Source: CAD feature listing. Evaluate the final solid. Frame: model axes, mm. A direction names the side the tool comes from. Round coordinates to 2 decimals unless told otherwise and drop trailing zeros. Loops run counter-clockwise (first coordinate to the right, second up) from the corner with the lowest first, then second, coordinate; pieces in that order, holes last. Notation, with made-up numbers: (-7, 30.25) - (34, 30.25) arc R11 ccw to (34, 39.25) - close; hole circle Ø6 at (70, -27.5). An arc over 180 degrees is marked (long way). Write item = value, one per line. Start each with the question number.
from build123d import *

# Parameters (mm, degrees)
SKETCH1_R           = 1.25
BOSS_EXTRUDE1_DEPTH = 2
SKETCH2_W           = 6
SKETCH2_H           = 2.8
BOSS_EXTRUDE2_DEPTH = 4
SKETCH3_R           = 1.25
BOSS_EXTRUDE3_DEPTH = 4
BOSS_EXTRUDE4_DEPTH = 2
CUT_EXTRUDE1_DEPTH  = 4


with BuildPart() as part:
    # Sketch1 → Boss-Extrude1 (new body)
    with BuildSketch(Plane.XY):
        with BuildLine():
            Line((-14.5, -1.25), (-3.25, -1.25))
            Line((-3.25, -1.25), (-3.25, 0))
            ThreePointArc((-3.25, 0), (0, 3.25), (3.25, 0))
            Line((3.25, 0), (3.25, -1.25))
            Line((3.25, -1.25), (7.5, -1.25))
            ThreePointArc((7.5, -1.25), (10, -3.75), (7.5, -6.25))
            Line((7.5, -6.25), (-14.5, -6.25))
            ThreePointArc((-14.5, -6.25), (-17, -3.75), (-14.5, -1.25))
        make_face()
        Circle(SKETCH1_R, mode=Mode.SUBTRACT)
    extrude(amount=BOSS_EXTRUDE1_DEPTH)

    # Sketch2 → Boss-Extrude2 (add)
    with BuildSketch(Plane.XY.offset(2)):
        with BuildLine():
            Line((-15, -6.199489743), (-15, -1.300510257))
            ThreePointArc((-15, -1.300510257), (-17, -3.75), (-15, -6.199489743))
        make_face()
        with Locations((0, -4.85)):
            Rectangle(SKETCH2_W, SKETCH2_H)
        with BuildLine():
            Line((8, -1.300510257), (8, -6.199489743))
            ThreePointArc((8, -6.199489743), (10, -3.75), (8, -1.300510257))
        make_face()
    extrude(amount=BOSS_EXTRUDE2_DEPTH)


with BuildPart() as body_2:
    # Sketch3 → Boss-Extrude3 (new body)
    with BuildSketch(Plane.XY.offset(2)):
        with BuildLine():
            Line((-3.25, 0), (-3.25, -3.25))
            Line((-3.25, -3.25), (-1.05, -3.25))
            Line((-1.05, -3.25), (-1.05, -6.25))
            Line((-1.05, -6.25), (1.05, -6.25))
            Line((1.05, -6.25), (1.05, -3.25))
            Line((1.05, -3.25), (3.25, -3.25))
            Line((3.25, -3.25), (3.25, 0))
            ThreePointArc((3.25, 0), (0, 3.25), (-3.25, 0))
        make_face()
        Circle(SKETCH3_R, mode=Mode.SUBTRACT)
    extrude(amount=BOSS_EXTRUDE3_DEPTH)

    # Sketch4 → Boss-Extrude4 (add)
    with BuildSketch(Plane.XY.offset(6)):
        with BuildLine():
            Line((7.5, -1.25), (3.25, -1.25))
            Line((3.25, -1.25), (3.25, 0))
            ThreePointArc((3.25, 0), (0, 3.25), (-3.25, 0))
            Line((-3.25, 0), (-3.25, -1.25))
            Line((-3.25, -1.25), (-14.5, -1.25))
            ThreePointArc((-14.5, -1.25), (-17, -3.75), (-14.5, -6.25))
            Line((-14.5, -6.25), (7.5, -6.25))
            ThreePointArc((7.5, -6.25), (10, -3.75), (7.5, -1.25))
        make_face()
    extrude(amount=BOSS_EXTRUDE4_DEPTH)

    # Sketch5 → Cut-Extrude1 (cut)
    with BuildSketch(Plane.XY.offset(8)):
        Polygon((1.154700538, 2), (-1.154700538, 2), (-2.309401077, 0), (-1.154700538, -2), (1.154700538, -2), (2.309401077, 0), align=None)
    extrude(amount=-CUT_EXTRUDE1_DEPTH, mode=Mode.SUBTRACT)


solid = body_2.part
(1) Cut plane C-C (y = -3.75). Output: boundary loops of the cut face in (x, z), and give its area (3 significant figures).
(2) Cut plane B-B (z = 5.2). Output: boundary loops of the cut face in (x, y), and give its area (3 significant figures).
(3) Material intervals for line 1 along Y through (x, z) = (0, 2.65); line 2 along Z through (x, y) = (-7, -4.75); line 3 along X through (y, z) = (-0.25, 3.8), sorted ascending. Write a range as from..to.
(4) Cut plane D-D (z = 7.45). Output: boundary loops of the cut face in (x, y), and give its area (3 significant figures).
(5) Pin query (flat end, axial travel): P1, Ø3, axis at x = 0.5, y = 0, coming from the +Z side; P2, Ø0.9, axis at y = -4.5, z = 4, coming from the +X side; P3, Ø1.6, axis at x = -10, z = 6.5, coming from the +Y side; P4, Ø1, axis at x = -9, z = 5, coming from the +Y side. Return the tip coordinate at first contact, or that it passes through.
(6) Cut plane A-A (x = 0.25). Output: boundary loops of the cut face in (y, z), and give its area (3 significant figures).
(7) Access query for faces 4 (the face through (-9, -1.25, 7)), 5 (the face through (-1.05, -5, 4)), 6 (the face through (1.05, -5, 4)), 7 (the face through (-1.74, -0.99, 6.03)). Directions: +Z, -Z, +X, -X, +Y, -Y. A direction counts if a zero-diameter tool reaches every point of the face in a straight line with its end or side. Return the directions, or none.
(8) Mould query, pull axis Y, two halves, no side actions, for faces 1 (the face through (1, 1, 4)), 2 (the face through (5, -4, 6)), 3 (the face through (-3, -6.25, 7)). Classes: +Y half, -Y half, draft (parallel to the pull), parting line (faces both ways), or undercut.
Solution:
q1.outline = (-17, 6) - (-1.05, 6) - (-1.05, 2) - (1.05, 2) - (1.05, 6) - (10, 6) - (10, 8) - (-17, 8) - close
q1.area = 62.4 mm^2
q2.outline = (-3.25, -3.25) - (-1.05, -3.25) - (-1.05, -6.25) - (1.05, -6.25) - (1.05, -3.25) - (3.25, -3.25) - (3.25, 0) arc R3.25 ccw to (-3.25, 0) - close; hole (-2.31, 0) - (-1.15, -2) - (1.15, -2) - (2.31, 0) - (1.15, 2) - (-1.15, 2) - close
q2.area = 30.2 mm^2
q3.line_1 = -6.25..-1.25, 1.25..3.25
q3.line_2 = 6..8
q3.line_3 = -3.25..-1.22, 1.22..3.25
q4.outline = (-14.5, -6.25) - (7.5, -6.25) arc R2.5 ccw to (7.5, -1.25) - (3.25, -1.25) - (3.25, 0) arc R3.25 ccw to (-3.25, 0) - (-3.25, -1.25) - (-14.5, -1.25) arc R2.5 ccw to start; hole (-2.31, 0) - (-1.15, -2) - (1.15, -2) - (2.31, 0) - (1.15, 2) - (-1.15, 2) - close
q4.area = 140 mm^2
q5.P1 = 4
q5.P2 = 1.05
q5.P3 = -1.25
q5.P4 = through
q6.outline = (-6.25, 2) - (-1.22, 2) - (-1.22, 4) - (-2, 4) - (-2, 8) - (-6.25, 8) - close; (1.22, 2) - (3.24, 2) - (3.24, 8) - (2, 8) - (2, 4) - (1.22, 4) - close
q6.area = 36.0 mm^2
q7.face_4 = +Z, -Z, -X, +Y
q7.face_5 = -Z, -X, -Y
q7.face_6 = -Z, +X, -Y
q7.face_7 = +Z
q8.face_1 = undercut
q8.face_2 = draft
q8.face_3 = -Y half
